Study the drawing (mm; zero at the part's minimum x, y, z) and answer. Round coordinates to 2 decimals unless told otherwise and drop trailing zeros. Write each loop counter-clockwise with the first axis right and the second up, starting at its lowest first coordinate (ties: lowest second). Pieces come first, ordered by that corner, then holes. Notation, with made-up numbers: M 28,35 L 53,35 A5 ccw 53,41 Z; hole C -1,7 d6. An arc over 180 degrees is marked long. Write each question's results on one line, items separated by ' | '.
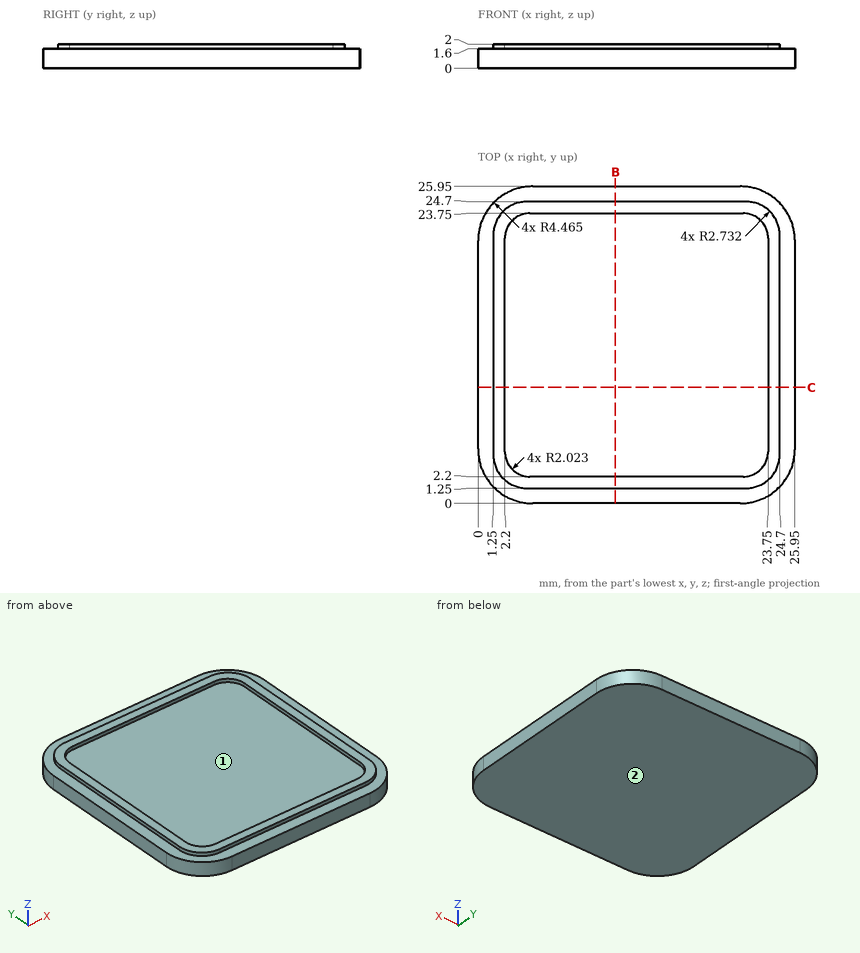
1) The mould has two halves that part along Y. Classify the marked faces 1 and 2: +Y half, -Y half, draft (parallel to the pull), parting line (faces both ways), or undercut.
Return value:
face 1: undercut | face 2: draft
2) Find the intervals of material crossed by line 1 (Z direction, x = 11, y = 11.5); line 2 (X direction, y = 21.75, z = 0.5); line 3 (X direction, y = 2.75, z = 1.65) (1 decimal), in increasing order.
Return value:
line 1: 0 to 1.6 | line 2: 0.01 to 25.94 | line 3: 1.5 to 2.8, 23.1 to 24.4
3) Section B-B (x = 11.25) is taken. Determine the outline of the cut face in (y, z).
Return value:
outline: M 0,0 L 25.95,0 L 25.95,1.6 L 24.7,1.6 L 24.7,2 L 23.75,2 L 23.75,1.6 L 2.2,1.6 L 2.2,2 L 1.25,2 L 1.25,1.6 L 0,1.6 Z
4) This flat-tipped pin is pushed along its axis until it touches: pin 1 (12 mm diameter, centred on x = 11, y = 13, fed in from +Z). Where does it stop, or does it pass through?
Return value:
pin 1: z = 1.6
